For this review, take the finished solid that the model builds, in its own axes (mm). A direction names the side the tool comes from. Round coordinates to 2 decimals unless told otherwise and drop trailing zeros. Loops run counter-clockwise (first coordinate to the right, second up) from the corner with the lowest first, then second, coordinate; pieces in that order, holes last.
1) Insertion check: pin 1 (2.5 mm diameter, centred on x = -45, z = 3, fed in from -Y). The pin has a flat end and moves straight along its axis. Give the tip position at first contact, or say it passes through.
2) Mouldability with a two-part tool opening along X and no side actions: class faces 4 (the flat face through (-264.805, -133.749, 2.465)), 5 (the flat face through (-124, 4, 0)), 6 (the cylindrical face through (28.021, -10.714, 2.465)) as pulls with the +X half, pulls with the -X half, needs draft (parallel to the pull), parting line crosses it, or undercut.
3) Wall thickness on L1, parallel to Y at x = -67, z = 1.65; L2, parallel to Y at x = -24, z = 2.7; L3, parallel to X at y = -14, z = 1.6: over which ranges is each line inside the solid? List them lowest first.
4) Tool access review of faces 1 (the flat face through (-182, -37, 2)), 2 (the flat face through (-28, -28, 2)), 3 (the flat face through (-173.372, -56.656, 2.465)): name each direction out of +Z, -Z, +X, -X, +Y, -Y from which nothing blocks a thin tool from reaching the whole face with its end or side.
5) Take a section at D-D (y = -94.5). State the section outline as (x, z) points.
6) Take a section at C-C (y = 9.5). State the section outline as (x, z) points, then the cut area to 3 significant figures.
7) Take a section at A-A (x = 10). State the section outline as (y, z) points.
8) Take a section at B-B (z = 1.8). State the section outline as (x, y) points.
```python
from build123d import *

# Parameters (mm, degrees)
EXTRUDE_1_DEPTH     = 5
SKETCH_2_R          = 1.5
CUT_EXTRUDE_1_DEPTH = 307.179177957


with BuildPart() as part:
    # 草图1 → 凸台-拉伸1 (new body)
    with BuildSketch(Plane.XY):
        with BuildLine():
            Line((0, 50), (-95, 50))
            Line((-95, 50), (-271.776695297, -126.776695297))
            Line((-271.776695297, -126.776695297), (-257.634559673, -140.91883092))
            Line((-257.634559673, -140.91883092), (-86.715728753, 30))
            Line((-86.715728753, 30), (0, 30))
            ThreePointArc((0, 30), (27.716385975, -11.480502971), (-21.213203436, -21.213203436))
            Line((-21.213203436, -21.213203436), (-35.355339059, -35.355339059))
            ThreePointArc((-35.355339059, -35.355339059), (46.193976626, -19.134171618), (0, 50))
        make_face()
    extrude(amount=EXTRUDE_1_DEPTH)

    # 草图2 → 切除-拉伸1 (cut, through all)
    with BuildSketch(Plane.XY.offset(5)):
        with Locations((-257.634559673, -126.776695297)):
            Circle(SKETCH_2_R)
        with Locations((-247.735064736, -116.87720036)):
            Circle(SKETCH_2_R)
    extrude(amount=-CUT_EXTRUDE_1_DEPTH, mode=Mode.SUBTRACT)


solid = part.part
```
Response:
1. pin 1: stops at y = 30
2. face 4: pulls with the -X half
2. face 5: needs draft
2. face 6: undercut
3. L1: y = 30 to 50
3. L2: y = -43.86 to -24, 30 to 50
3. L3: x = -159 to -130.72, 26.53 to 48
4. face 1: +Z, -Z, -X, +Y
4. face 2: +Z, -Z
4. face 3: +Z, -Z, -Y
5. outline: (-239.5, 0) - (-211.22, 0) - (-211.22, 5) - (-239.5, 5) - close
6. outline: (-135.5, 0) - (-107.22, 0) - (-107.22, 5) - (-135.5, 5) - close; (28.46, 0) - (49.09, 0) - (49.09, 5) - (28.46, 5) - close
6. area: 245 mm2
7. outline: (-48.99, 0) - (-28.28, 0) - (-28.28, 5) - (-48.99, 5) - close; (28.28, 0) - (48.99, 0) - (48.99, 5) - (28.28, 5) - close
8. outline: (-271.78, -126.78) - (-257.63, -140.92) - (-86.72, 30) - (0, 30) arc R30 cw (long way) to (-21.21, -21.21) - (-35.36, -35.36) arc R50 ccw (long way) to (0, 50) - (-95, 50) - close; hole circle Ø3 at (-257.63, -126.78); hole circle Ø3 at (-247.74, -116.88)
